Read the model definition and answer for the solid it produces. Units are mm, in the model's axes. A direction names the side the tool comes from. Round coordinates to 2 decimals unless told otherwise and drop trailing zeros. Loops run counter-clockwise (first coordinate to the right, second up) from the corner with the lowest first, then second, coordinate; pieces in that order, holes last. Notation, with made-up numbers: (9, -15) - (53, -15) arc R23 cw to (53, -1) - close; hole circle Ø4 at (25.25, 14). An arc over 180 degrees is marked (long way). Answer as CSV lines item,"result".
```python
from build123d import *

# Parameters (mm, degrees)
SKETCH1_R             = 5.953125
BOSS_EXTRUDE1_DEPTH   = 1.778
BOSS_EXTRUDE2_DEPTH   = 3.381375
F_8_32_TAPPED_HOLE1_D = 3.4544
CHAMFER1_SIZE         = 0.254


with BuildPart() as part:
    # Sketch1 → Boss-Extrude1 (new body)
    with BuildSketch(Plane(origin=(0, 0, 0), x_dir=(1, 0, 0), z_dir=(0, 1, 0))):
        Circle(SKETCH1_R)
    extrude(amount=BOSS_EXTRUDE1_DEPTH)

    # Sketch2 → Boss-Extrude2 (add)
    with BuildSketch(Plane(origin=(0, 1.778, 0), x_dir=(1, 0, 0), z_dir=(0, 1, 0))):
        Polygon((4.365625, -2.520494769), (4.365625, 2.520494769), (0, 5.040989538), (-4.365625, 2.520494769), (-4.365625, -2.520494769), (0, -5.040989538), align=None)
    extrude(amount=BOSS_EXTRUDE2_DEPTH)

    # #8-32 Tapped Hole1 (through all)
    with Locations(Plane(origin=(0, 5.159375, 0), x_dir=(1, 0, 0), z_dir=(0, 1, 0))):
        with Locations((0, 0)):
            Hole(F_8_32_TAPPED_HOLE1_D / 2)

    # Chamfer1
    chamfer1_edges = [part.edges().sort_by_distance(p)[0] for p in [
        (-5.953125, 0, 0),
        (1.7272, 5.159375, 0),
        (1.7272, 0, 0),
        (-5.953125, 1.778, 0),
    ]]
    chamfer(chamfer1_edges, length=CHAMFER1_SIZE)


solid = part.part
```
1) The mould has two halves that part along X. Classify faces 1 (the face through (2.213, 3.445, -3.763)), 2 (the face through (3, 1.778, 4)), 3 (the face through (0.225, 2.547, -1.713)): pulls with the +X half, pulls with the -X half, needs draft (parallel to the pull), parting line crosses it, or undercut.
Entries:
face 1,"pulls with the +X half"
face 2,"needs draft"
face 3,"undercut"
2) Each of these flat-tipped pins is pushed along its axis until it touches: P1, Ø2.5, axis at y = 3.5, z = 1, coming from the -X side; P2, Ø1.5, axis at y = 3.5, z = 4, coming from the +X side; P3, Ø6, axis at x = 4, z = -3.5, coming from the -Y side; P4, Ø2, axis at x = -1.5, y = 4.5, coming from the -Z side. Where does it stop, or does it pass through?
Entries:
P1,"stops at x = -4.37"
P2,"stops at x = 3.1"
P3,"stops at y = 0"
P4,"stops at z = -4.75"
3) A cutting plane is placed at A-A, the plane z = 0. Determine the outline of the cut face in (x, y), plus the area to 3 significant figures.
Entries:
outline,"(-5.95, 0.25) - (-5.7, 0) - (-1.98, 0) - (-1.73, 0.25) - (-1.73, 4.91) - (-1.98, 5.16) - (-4.37, 5.16) - (-4.37, 1.78) - (-5.7, 1.78) - (-5.95, 1.52) - close; (1.73, 0.25) - (1.98, 0) - (5.7, 0) - (5.95, 0.25) - (5.95, 1.52) - (5.7, 1.78) - (4.37, 1.78) - (4.37, 5.16) - (1.98, 5.16) - (1.73, 4.91) - close"
area,"32.6 mm^2"
4) A tool of negligible diameter and unlimited length cuts with its end or side. For faces 4 (the face through (-2.15, 3.45, -3.8)), 5 (the face through (-2.213, 3.445, 3.763)), 6 (the face through (-4.366, 3, 0)), from which of +Z, -Z, +X, -X, +Y, -Y can it reach the whole face along a straight path? Write none if from no direction.
Entries:
face 4,"-Z, -X, +Y"
face 5,"+Z, -X, +Y"
face 6,"+Z, -Z, -X, +Y"
5) A cutting plane is placed at B-B, the plane y = 4.3. Determine the outline of the cut face in (x, z), plus the area to 3 significant figures.
Entries:
outline,"(-4.37, -2.52) - (0, -5.04) - (4.37, -2.52) - (4.37, 2.52) - (0, 5.04) - (-4.37, 2.52) - close; hole circle Ø3.45 at (0, 0)"
area,"56.6 mm^2"
6) Find the intervals of material crossed by line 1 (X direction, y = 1.45, z = 0); line 2 (X direction, y = 2.55, z = 0), in increasing order.
Entries:
line 1,"x = -5.95 to -1.73, 1.73 to 5.95"
line 2,"x = -4.37 to -1.73, 1.73 to 4.37"
